from build123d import *

# Parameters (mm, degrees)
BOSS_EXTRUDE1_DEPTH = 11.1252
SKETCH5_R           = 17.4625
CUT_EXTRUDE1_DEPTH  = 12.7
CUT_EXTRUDE4_DEPTH  = 12.7
BOSS_EXTRUDE2_DEPTH = 6.35


# Read off the part's stored shape, not the designer's step: Boss-Extrude2
with BuildPart() as part:
    # Sketch1 → Boss-Extrude1 (new body)
    with BuildSketch(Plane.XY):
        with BuildLine():
            Line((37.67911766, 180.254005759), (37.601979843, 213.274005759))
            Line((37.601979843, 213.274005759), (-38.598020157, 213.095995412))
            Line((-38.598020157, 213.095995412), (-38.52088234, 180.075995412))
            ThreePointArc((-38.52088234, 180.075995412), (-184.15, 0), (-38.52088234, -180.075995412))
            Line((-38.52088234, -180.075995412), (-38.52088234, -211.825995412))
            Line((-38.52088234, -211.825995412), (37.67911766, -211.825995412))
            Line((37.67911766, -211.825995412), (37.67911766, -180.254005759))
            ThreePointArc((37.67911766, -180.254005759), (184.15, 0), (37.67911766, 180.254005759))
        make_face()
    extrude(amount=BOSS_EXTRUDE1_DEPTH)

    # Sketch5 → Cut-Extrude1 (cut)
    with BuildSketch(Plane.XY.offset(11.1252)):
        Circle(SKETCH5_R)
    extrude(amount=-CUT_EXTRUDE1_DEPTH, mode=Mode.SUBTRACT)

    # Sketch6 → Cut-Extrude4 (cut)
    with BuildSketch(Plane.XY.offset(11.1252)):
        with BuildLine():
            ThreePointArc((90.375326038, -138.167689579), (0, -29.126312042), (-90.375326038, -138.167689579))
            ThreePointArc((-90.375326038, -138.167689579), (0, -165.1), (90.375326038, -138.167689579))
        make_face()
    extrude(amount=-CUT_EXTRUDE4_DEPTH, mode=Mode.SUBTRACT)

    # Boss-Extrude2 outline → Boss-Extrude2 (add)
    with BuildSketch(Plane.XY.offset(11.1252)):
        with BuildLine():
            ThreePointArc((34.149976763, -161.529530078), (-2.240394082, -165.084798314), (-38.52088234, -160.543301398))
            Line((-38.52088234, -160.543301398), (-38.52088234, -180.075995412))
            Line((-38.52088234, -180.075995412), (34.149976763, -180.075995412))
            Line((34.149976763, -180.075995412), (34.149976763, -161.529530078))
        make_face()
    extrude(amount=BOSS_EXTRUDE2_DEPTH)


solid = part.part
Check sheet for the modelled part. Datum: model origin and axes. Units: mm. A direction names the side the tool comes from. Round coordinates to 2 decimals unless told otherwise and drop trailing zeros. Order: outer loops, then holes, each group sorted by start corner. A loop starts at its lowest first (then second) coordinate and runs counter-clockwise, first axis right, second up.
Q1. Scan lines: L1, parallel to Y at x = 0, z = 6.5; L2, parallel to Z at x = -87, y = -76; L3, parallel to X at y = -84.5, z = 9. Record each from-to range of solid material in increasing order.
Filled sheet:
L1: y = -211.83 to -165.1, -29.13 to -17.46, 17.46 to 213.19
L2: z = 0 to 11.13
L3: x = -163.62 to -84.38, 84.38 to 163.62
Q2. Cross-section at B-B, the plane y = 0. Enter the section's corners in (x, z).
Filled sheet:
outline: (-184.15, 0) - (-17.46, 0) - (-17.46, 11.13) - (-184.15, 11.13) - close; (17.46, 0) - (184.15, 0) - (184.15, 11.13) - (17.46, 11.13) - close
Q3. Cross-section at C-C, the plane x = 76. Enter the section's corners in (y, z), plus the area to 3 significant figures.
Filled sheet:
outline: (-167.74, 0) - (-146.57, 0) - (-146.57, 11.13) - (-167.74, 11.13) - close; (-69.3, 0) - (167.74, 0) - (167.74, 11.13) - (-69.3, 11.13) - close
area: 2,870 mm2
Q4. Draft check along X on faces 3 (the face through (37.679, -196, 5)), 4 (the face through (-3, 51, 11.125)), 5 (the face through (-13.858, -10.626, 5.64)). Enter one of: pulls with the +X half, pulls with the -X half, needs draft (parallel to the pull), parting line crosses it, or undercut.
Filled sheet:
face 3: pulls with the +X half
face 4: needs draft
face 5: undercut
Q5. Set-up check for faces 1 (the face through (-38.521, -196, 5)), 2 (the face through (-1, -211.826, 5)): record each of +Z, -Z, +X, -X, +Y, -Y from which the full face is reachable in a straight line by a thin tool's end or side.
Filled sheet:
face 1: +Z, -Z, -X, -Y
face 2: +Z, -Z, +X, -X, -Y
Q6. Cross-section at A-A, the plane z = 6. Give the number of separate pieces and of enclosed holes in the cut face, plus the area to 3 significant figures.
Filled sheet:
separate pieces: 1
enclosed holes: 2
area: 90,400 mm2
Q7. Cross-section at D-D, the plane x = 0. Enter the section's corners in (y, z), plus the area to 3 significant figures.
Filled sheet:
outline: (-211.83, 0) - (-165.1, 0) - (-165.1, 17.48) - (-180.08, 17.48) - (-180.08, 11.13) - (-211.83, 11.13) - close; (-29.13, 0) - (-17.46, 0) - (-17.46, 11.13) - (-29.13, 11.13) - close; (17.46, 0) - (213.19, 0) - (213.19, 11.13) - (17.46, 11.13) - close
area: 2,920 mm2
Q8. Depth check by flat-ended pin: P1, Ø8, axis at x = 81, z = 14, coming from the -Y side; P2, Ø2, axis at x = 134.5, y = -96, coming from the +Z side; P3, Ø5, axis at x = -19.5, z = 15, coming from the -Y side; P4, Ø4, axis at x = 98.5, y = 23.5, coming from the -Z side. Enter the tip coordinate at first touch or a pass-through.
Filled sheet:
P1: stops at y = -166.71
P2: stops at z = 11.13
P3: stops at y = -180.08
P4: stops at z = 0
